from build123d import *

# Parameters (mm, degrees)
BOSS_EXTRUDE1_DEPTH = 1
BOSS_EXTRUDE2_DEPTH = 5
FILLET1_R           = 2
BOSS_EXTRUDE3_DEPTH = 15.95
SKETCH10_R          = 4.5
SKETCH10_R_2        = 3.5
BOSS_EXTRUDE7_DEPTH = 2.33
CUT_EXTRUDE1_START  = -1
SKETCH13_R          = 3.5
CUT_EXTRUDE1_DEPTH  = 1


with BuildPart() as part:
    # Sketch1 → Boss-Extrude1 (new body)
    with BuildSketch(Plane.XY):
        Polygon((86.661024886, 23.401143993), (29.430818123, 23.401143993), (42.074789018, 1.501143993), (74.017053991, 1.501143993), align=None)
    extrude(amount=BOSS_EXTRUDE1_DEPTH)

    # Sketch2 → Boss-Extrude2 (add)
    with BuildSketch(Plane(origin=(0, 0, 0), x_dir=(-1, 0, 0), z_dir=(0, 0, -1))):
        Polygon((-74.017053991, 1.501143993), (-71.117053991, 1.501143993), (-71.117053991, 7.401143993), (-77.423420579, 7.401143993), align=None)
        Polygon((-42.074789018, 1.501143993), (-44.974789018, 1.501143993), (-44.974789018, 7.401143993), (-38.66842243, 7.401143993), align=None)
    extrude(amount=BOSS_EXTRUDE2_DEPTH)

    # Fillet1
    # the kernel refuses this fillet: 2 mm, written as the material it takes off along each edge
    with BuildSketch(Plane(origin=(44.974789018, -3.498856007, -5), x_dir=(-1, 0, 0), z_dir=(0, 1, 0)), Plane(origin=(71.117053991, -3.498856007, -5), x_dir=(0, 0, 1), z_dir=(0, 1, 0))) as fillet1_piece_1:
        with BuildLine():
            CenterArc((FILLET1_R, FILLET1_R), FILLET1_R, 180, 90)
            Line((0, FILLET1_R), (0, 0))
            Line((0, 0), (FILLET1_R, 0))
        make_face()
    extrude(amount=15.9, mode=Mode.SUBTRACT)
    with BuildSketch(Plane(origin=(49.974789018, 7.401143993, -5), x_dir=(0, -1, 0), z_dir=(-1, 0, 0)), Plane(origin=(66.117053991, 7.401143993, -5), x_dir=(0, 0, 1), z_dir=(1, 0, 0))) as fillet1_piece_2:
        with BuildLine():
            CenterArc((FILLET1_R, FILLET1_R), FILLET1_R, 180, 90)
            Line((0, FILLET1_R), (0, 0))
            Line((0, 0), (FILLET1_R, 0))
        make_face()
    extrude(amount=16.306366588, mode=Mode.SUBTRACT)
    with BuildSketch(Plane(origin=(36.16842243, 11.731271012, -5), x_dir=(0.8660254037844386, 0.5000000000000002, 0), z_dir=(0.5000000000000002, -0.8660254037844386, 0))) as fillet1_piece_3:
        with BuildLine():
            CenterArc((FILLET1_R, FILLET1_R), FILLET1_R, 180, 90)
            Line((0, FILLET1_R), (0, 0))
            Line((0, 0), (FILLET1_R, 0))
        make_face()
    extrude(amount=16.812733176, mode=Mode.SUBTRACT)
    with BuildSketch(Plane(origin=(79.923420579, 11.731271012, -5), x_dir=(-0.866025403784438, 0.500000000000001, 0), z_dir=(-0.500000000000001, -0.8660254037844382, 0))) as fillet1_piece_4:
        with BuildLine():
            CenterArc((FILLET1_R, -FILLET1_R), FILLET1_R, 90, 90)
            Line((0, -FILLET1_R), (0, 0))
            Line((0, 0), (FILLET1_R, 0))
        make_face()
    extrude(amount=16.812733176, mode=Mode.SUBTRACT)

    # Sketch4 → Boss-Extrude3 (add)
    with BuildSketch(Plane.XY.offset(1)):
        Polygon((42.190259072, 1.501143993), (73.901583937, 1.501143993), (86.545554832, 23.401143993), (84.545554832, 23.401143993), (72.439703722, 2.501143993), (43.652139287, 2.501143993), (31.585518661, 23.401143993), (29.546288176, 23.401143993), align=None)
    extrude(amount=BOSS_EXTRUDE3_DEPTH)

    # Sketch10 → Boss-Extrude7 (add)
    with BuildSketch(Plane(origin=(0, 2.501143993, 0), x_dir=(1, 0, 0), z_dir=(0, 1, 0))):
        with Locations((58.045921504, -11)):
            Circle(SKETCH10_R)
        with Locations(Location((58.045921504, -11, 0), (0, 0, 180))):
            Circle(SKETCH10_R_2, mode=Mode.SUBTRACT)
    extrude(amount=BOSS_EXTRUDE7_DEPTH)

    # Sketch13 → Cut-Extrude1 (cut)
    with BuildSketch(Plane(origin=(0, 2.501143993, 0), x_dir=(1, 0, 0), z_dir=(0, 1, 0)).offset(CUT_EXTRUDE1_START)):
        with Locations(Location((58.045921504, -11, 0), (0, 0, 180))):
            Circle(SKETCH13_R)
    extrude(amount=CUT_EXTRUDE1_DEPTH, mode=Mode.SUBTRACT)


solid = part.part
Input: part model. Units: mm. Frame: model coordinates. A direction names the side the tool comes from. Give positions to 0.01 mm unless a question says otherwise; leave off trailing zeros. Order: outer loops, then holes, each group sorted by start corner. A loop starts at its lowest first (then second) coordinate and runs counter-clockwise, first axis right, second up.
Q1. Section D-D on z = 2.75. Output: boundary loops of the cut face in (x, y).
Checked values:
outline: (29.55, 23.4) - (42.19, 1.5) - (73.9, 1.5) - (86.55, 23.4) - (84.55, 23.4) - (72.44, 2.5) - (43.65, 2.5) - (31.59, 23.4) - close
Q2. Section C-C on y = 10.5. Output: boundary loops of the cut face in (x, z).
Checked values:
outline: (36.88, 0) - (79.21, 0) - (79.21, 1) - (79.1, 1) - (79.1, 16.95) - (77.07, 16.95) - (77.07, 1) - (39.03, 1) - (39.03, 16.95) - (36.99, 16.95) - (36.99, 1) - (36.88, 1) - close
Q3. Contact query for flat-ended pins moving along their axis: pin 1 Ø6.5 at (x, y) = (80, 11) entering from +Z; pin 2 Ø10 at (x, z) = (57, 10) entering from +Y; pin 3 Ø2 at (y, z) = (17, 0) entering from +X; pin 4 Ø5 at (x, y) = (55, 16.5) entering from -Z. Output: stop coordinate, or through.
Checked values:
pin 1: stops at z = 16.95
pin 2: stops at y = 4.83
pin 3: stops at x = 83.54
pin 4: stops at z = 0
Q4. Draft query along X for faces 1 (the flat face through (78.58, 13.1, 8.86)), 2 (the cylindrical face through (75.228, 4.348, -4.165)), 3 (the flat face through (58, 15, 1)), 4 (the flat face through (35.78, 12.604, 8.863)). Return one class per face: +X half, -X half, draft (parallel to the pull), parting line (faces both ways), or undercut.
Checked values:
face 1: undercut
face 2: +X half
face 3: undercut
face 4: -X half
Q5. Section B-B on x = 53. Output: boundary loops of the cut face in (y, z).
Checked values:
outline: (1.5, 0) - (23.4, 0) - (23.4, 1) - (2.5, 1) - (2.5, 16.95) - (1.5, 16.95) - close
Q6. Section A-A on z = 11. Output: boundary loops of the cut face in (x, y), and give its area (3 significant figures).
Checked values:
outline: (29.55, 23.4) - (42.19, 1.5) - (54.55, 1.5) - (54.55, 4.83) - (53.55, 4.83) - (53.55, 2.5) - (43.65, 2.5) - (31.59, 23.4) - close; (61.55, 1.5) - (73.9, 1.5) - (86.55, 23.4) - (84.55, 23.4) - (72.44, 2.5) - (62.55, 2.5) - (62.55, 4.83) - (61.55, 4.83) - close
area: 115 mm2
Q7. Set-up query: faces 5 (the flat face through (80.135, 12.298, 8.863)), 6 (the cylindrical face through (62.34, 3.65, 9.65)), 7 (the cylindrical face through (71.491, 4.41, -4.165)). Return all of +Z, -Z, +X, -X, +Y, -Y with unobstructed straight access to the full face (end or side cutting, diameter ignored); none if empty.
Checked values:
face 5: +Z, +X, -Y
face 6: +Y
face 7: -Z, +Y, -Y
Q8. Ray query, probe 1 along Z at (x, y) = (70.5, 17.75); probe 2 along Y at (x, z) = (57.5, 6.25); probe 3 along X at (y, z) = (18, 3.75). Return the intervals inside material, ascending.
Checked values:
probe 1: z = 0 to 1
probe 2: y = 1.5 to 2.5
probe 3: x = 32.66 to 34.7, 81.42 to 83.43
